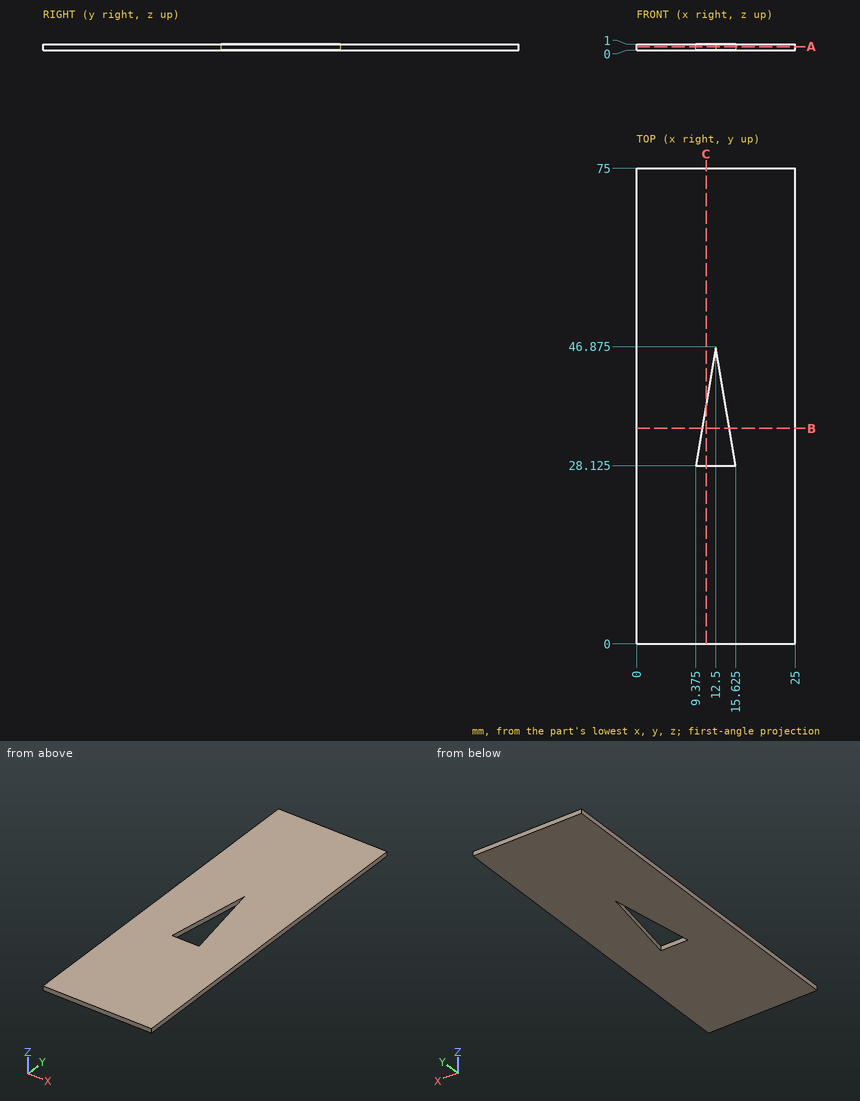
Drawing for the job (mm, zero at the part's lowest x, y, z). Give positions to 0.01 mm unless a question says otherwise; leave off trailing zeros. Loops run counter-clockwise (first coordinate to the right, second up) from the corner with the lowest first, then second, coordinate; pieces in that order, holes last.
(1) Drill centre lines: line 1 along X through (y, z) = (38, 0.7); line 2 along X through (y, z) = (42, 0.65). Where is each one in solid material? Low to high.
Return value:
line 1: x = 0 to 11.02, 13.98 to 25
line 2: x = 0 to 11.69, 13.31 to 25
(2) Band-saw the part on C-C (x = 11). Write the cut outline in (y, z) (3 decimals).
Return value:
outline: (0, 0) - (28.125, 0) - (28.125, 1) - (0, 1) - close; (37.875, 0) - (75, 0) - (75, 1) - (37.875, 1) - close
(3) Pin check, flat tip, straight feed: pin 1 (4 mm diameter, centred on x = 5.5, y = 45.5, fed in from -Z). Stop position of the tip, or through.
Return value:
pin 1: stops at z = 0
(4) Band-saw the part on B-B (y = 34). Write the cut outline in (x, z), and give its area (3 significant figures).
Return value:
outline: (0, 0) - (10.35, 0) - (10.35, 1) - (0, 1) - close; (14.65, 0) - (25, 0) - (25, 1) - (14.65, 1) - close
area: 20.7 mm2
(5) Band-saw the part on A-A (z = 0.6). Write the cut outline in (x, y) (3 decimals).
Return value:
outline: (0, 0) - (25, 0) - (25, 75) - (0, 75) - close; hole (9.375, 28.125) - (15.625, 28.125) - (12.5, 46.875) - close
